Input: part model. Units: mm. Frame: model coordinates. Face numbers are marked on the shaded views. A direction names the side the tool comes from. Round coordinates to 2 decimals unless told otherwise and drop trailing zeros. Return JSON: item names as keys, results as strings. Group by question number.
1) Contact query for flat-ended pins moving along their axis: P1, Ø7.5, axis at x = 7.5, y = 44, coming from the +Z side; P2, Ø20.5, axis at x = 12, y = 36.5, coming from the -Z side; P3, Ø10, axis at x = -25.5, z = 59, coming from the -Y side. Output: stop coordinate, or through.
2) Material intervals for line 1 (X direction, y = 42, z = 42); line 2 (X direction, y = 20, z = 15); line 3 (Z direction, x = -33, y = 7), sorted ascending. Write a range as from..to.
3) Access query for the marked faces 1, 2, 3, 4 and 5. Directions: +Z, -Z, +X, -X, +Y, -Y. A direction counts if a zero-diameter tool reaches every point of the face in a straight line with its end or side. Return the directions, or none.
from build123d import *

# Parameters (mm, degrees)
F0_W     = 25.4
F0_H     = 25.4
F1_DEPTH = 76.2
F2_W     = 25.4
F2_H     = 25.4
F3_DEPTH = 50.8
F4_W     = 25.4
F4_H     = 25.4
F5_DEPTH = 25.4
F6_R     = 25.39999


# Not quite as in the source:
# - a fillet or chamfer is up to 0.001 mm smaller than in the source, because OpenCascade refuses the exact size


with BuildPart() as f1:
    # F0 (on Top) → F1 (new body)
    with BuildSketch(Plane.XY):
        with Locations((12.7, 12.7)):
            Rectangle(F0_W, F0_H)
    extrude(amount=F1_DEPTH)

    # F2 (on face) → F3 (join)
    with BuildSketch(Plane(origin=(0, 0, 0), x_dir=(0, -1, 0), z_dir=(-1, 0, 0))):
        with Locations((-12.7, 63.5)):
            Rectangle(F2_W, F2_H)
    extrude(amount=F3_DEPTH)

    # F4 (on face) → F5 (join)
    with BuildSketch(Plane(origin=(0, 25.4, 0), x_dir=(-1, 0, 0), z_dir=(0, 1, 0))):
        with Locations((-12.7, 38.1)):
            Rectangle(F4_W, F4_H)
    extrude(amount=F5_DEPTH)

    # F6 (radius 25.4 in the source; OpenCascade refuses exactly that, so slightly less here)
    f6_edges = [f1.edges().sort_by_distance(p)[0] for p in [
        (-50.8, 12.7, 76.2),
        (-50.8, 0, 63.5),
        (-12.7, 0, 76.2),
        (25.4, 0, 38.1),
        (25.4, 12.7, 0),
        (12.7, 0, 0),
        (25.4, 12.7, 76.2),
    ]]
    fillet(f6_edges, radius=F6_R)


solid = f1.part
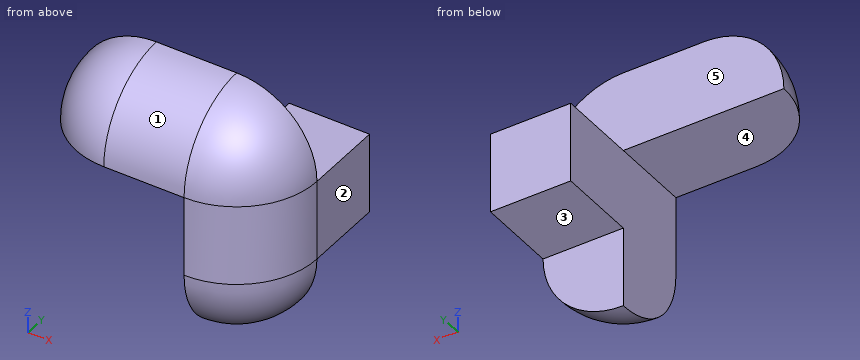
Returned:
{
 "1": {"P1": "stops at z = 50.8", "P2": "stops at z = 25.4", "P3": "stops at y = 0.2"},
 "2": {"line 1": "x = 0..25.4", "line 2": "x = 0..22.54", "line 3": "z = 50.8..66.57"},
 "3": {"face 1": "+Z, +X, -X, -Y", "face 2": "+Z, -Z, +X, +Y, -Y", "face 3": "-Z, +X, -X, +Y", "face 4": "-Z, -X, +Y, -Y", "face 5": "+Z, +X, -X, +Y"}
}
